from build123d import *

# Parameters (mm, degrees)
F0_R     = 43.18
F0_R_2   = 25.4
F1_DEPTH = 5.08
F2_DEPTH = 36.83
F6_R     = 5.08
F7_DEPTH = 2.54


# Not quite as in the source:
# - a fillet or chamfer that OpenCascade refuses, or shapes differently, is made with other operations: its cross-section is extruded or revolved along the edge and cut away or added


with BuildPart() as f1:
    # F0 (on Top) → F1 (new body)
    with BuildSketch(Plane.XY):
        Circle(F0_R)
        Circle(F0_R_2, mode=Mode.SUBTRACT)
    extrude(amount=F1_DEPTH)

    # F0 (on Top) → F2 (join)
    with BuildSketch(Plane.XY):
        Circle(F0_R_2)
    extrude(amount=F2_DEPTH)

    # F3 (on Front) → F4 (revolve)
    with BuildSketch(Plane.XZ):
        Polygon((0, 58.42), (0, 36.8297025561), (25.3384895623, 36.7359854281), (22.0302641392, 45.9328517318), (19.5160117, 50.1673817635), (16.4724439383, 54.8650622368), (11.0508995131, 58.42), align=None)
    revolve(axis=Axis((0, 0, 47.6248512781), (0, 0, 1)))

    # F5: fillet of radius 12.7 on 5 edges, made by hand

    # F5_s1 → F5_t2 (revolve, cut)
    with BuildSketch(Plane.XZ):
        with BuildLine():
            ThreePointArc((25.4, 35.2768549118), (25.3761454392, 36.0548888463), (25.3046713696, 36.83))
            Line((25.3046713696, 36.83), (25.4, 36.83))
            Line((25.4, 36.83), (25.4, 35.2768549118))
        make_face()
    revolve(axis=Axis((0, 0, 36.83), (0, 0, 1)), mode=Mode.SUBTRACT)

    # F5_s3 → F5_t4 (revolve, cut)
    with BuildSketch(Plane.XZ):
        with BuildLine():
            ThreePointArc((19.6427134925, 49.9539892906), (19.513951513, 50.166103437), (19.3810699459, 50.3756614184))
            Line((19.3810699459, 50.3756614184), (19.5160117, 50.1673817635))
            Line((19.5160117, 50.1673817635), (19.6427134925, 49.9539892906))
        make_face()
    revolve(axis=Axis((0, 0, 50.1673817635), (0, 0, 1)), mode=Mode.SUBTRACT)

    # F5_s5 → F5_t6 (revolve, cut)
    with BuildSketch(Plane.XZ):
        with BuildLine():
            ThreePointArc((22.4409800917, 44.79106143), (21.9779508662, 45.9081881165), (21.4107694035, 46.9762111901))
            Line((21.4107694035, 46.9762111901), (22.0302641392, 45.9328517318))
            Line((22.0302641392, 45.9328517318), (22.4409800917, 44.79106143))
        make_face()
    revolve(axis=Axis((0, 0, 45.9328517318), (0, 0, 1)), mode=Mode.SUBTRACT)

    # F5_s7 → F5_t8 (revolve, cut)
    with BuildSketch(Plane.XZ):
        with BuildLine():
            ThreePointArc((17.9281816755, 52.6181627827), (16.274530798, 54.6682321185), (14.2335662066, 56.3331072017))
            Line((14.2335662066, 56.3331072017), (16.4724439383, 54.8650622368))
            Line((16.4724439383, 54.8650622368), (17.9281816755, 52.6181627827))
        make_face()
    revolve(axis=Axis((0, 0, 54.8650622368), (0, 0, 1)), mode=Mode.SUBTRACT)

    # F5_s9 → F5_t10 (revolve, cut)
    with BuildSketch(Plane.XZ):
        with BuildLine():
            ThreePointArc((14.2223539104, 56.3404591686), (10.8923380013, 57.8890145748), (7.2584579428, 58.42))
            Line((7.2584579428, 58.42), (11.0508995131, 58.42))
            Line((11.0508995131, 58.42), (14.2223539104, 56.3404591686))
        make_face()
    revolve(axis=Axis((0, 0, 58.42), (0, 0, 1)), mode=Mode.SUBTRACT)

    # F6 (on face) → F7 (cut)
    with BuildSketch(Plane.XY.offset(58.42)):
        Circle(F6_R)
    extrude(amount=-F7_DEPTH, mode=Mode.SUBTRACT)


solid = f1.part
Read the model definition and answer for the solid it produces. Units are mm, in the model's axes. A direction names the side the tool comes from. Round coordinates to 2 decimals unless told otherwise and drop trailing zeros. Write each loop counter-clockwise with the first axis right and the second up, starting at its lowest first coordinate (ties: lowest second). Pieces come first, ordered by that corner, then holes. Notation, with made-up numbers: M -18,-22 L 22,-22 A27 cw 22,11 Z; hole C 33,-36 d4. An arc over 180 degrees is marked long. Use a Markdown table: item, result.
1) The part is cut by section A-A (x = 36). Write down the section's boundary in (y, z), plus the area to 3 significant figures.
Answers follow:
| item | result |
|---|---|
| outline | M -23.84,0 L 23.84,0 L 23.84,5.08 L -23.84,5.08 Z |
| area | 242 mm2 |
2) Straight lines are drawn through the part: line 1 along Z through (x, y) = (12.5, -26.5); line 2 along Z through (x, y) = (-2, -13.5); line 3 along Y through (x, z) = (0, 57). For each, find the intervals that lie inside material, in ascending order. Write a range as [from, to].
Answers follow:
| item | result |
|---|---|
| line 1 | z = [0, 5.08] |
| line 2 | z = [0, 56.7] |
| line 3 | y = [-13.09, -5.08], [5.08, 13.09] |
3) The part is cut by section B-B (z = 10). Write down the section's boundary in (x, y), plus the area to 3 significant figures.
Answers follow:
| item | result |
|---|---|
| outline | C 0,0 d50.8 |
| area | 2,030 mm2 |
4) The part is cut by section C-C (y = -36.5). Write down the section's boundary in (x, z), plus the area to 3 significant figures.
Answers follow:
| item | result |
|---|---|
| outline | M -23.07,0 L 23.07,0 L 23.07,5.08 L -23.07,5.08 Z |
| area | 234 mm2 |
5) A tool of negligible diameter and unlimited length cuts with its end or side. For faces 1 (the flat face through (2, 5, 58.42)), 2 (the flat face through (19, -19, 5.08)), from which of +Z, -Z, +X, -X, +Y, -Y can it reach the whole face along a straight path? Write none if from no direction.
Answers follow:
| item | result |
|---|---|
| face 1 | +Z, +X, -X, +Y, -Y |
| face 2 | +Z |
6) For a pull along X with two mould halves and no side action, classify faces 3 (the cylindrical face through (-0.661, 5.037, 57.168)), 4 (the flat face through (-1, 1, 0)), 5 (the flat face through (0, 0, 55.88)), 6 (the cylindrical face through (-5.506, -24.796, 19.967)) as pulls with the +X half, pulls with the -X half, needs draft (parallel to the pull), parting line crosses it, or undercut.
Answers follow:
| item | result |
|---|---|
| face 3 | undercut |
| face 4 | needs draft |
| face 5 | undercut |
| face 6 | parting line crosses it |
7) Flat-ended cylindrical pins translate along their axes: pin 1 (3 mm diameter, centred on y = -17, z = 51.5, fed in from -X); pin 2 (1 mm diameter, centred on y = -1.5, z = 26, fed in from -X); pin 3 (10 mm diameter, centred on x = -16, y = -1, fed in from +Z). Find the tip coordinate at first contact, or state that the pin passes through.
Answers follow:
| item | result |
|---|---|
| pin 1 | stops at x = -10.97 |
| pin 2 | stops at x = -25.38 |
| pin 3 | stops at z = 57.85 |
